Read the model definition and answer for the solid it produces. Units are mm, in the model's axes. Round coordinates to 2 decimals unless told otherwise and drop trailing zeros. Order: outer loops, then holes, each group sorted by start corner. A loop starts at its lowest first (then second) coordinate and runs counter-clockwise, first axis right, second up. Notation, with made-up numbers: M -7,7 L 9,7 A18 cw 9,12 Z; hole C -12.5,23.25 d1. An arc over 180 degrees is marked long. Use one line per item in the form item = value. Start each with the question number.
Autodesk Inventor part; units mm, degrees
ref_plane "YZ Plane" through (0, 0, 0) normal (1, 0, 0) x (0, 1, 0)
ref_plane "XZ Plane" through (0, 0, 0) normal (0, 1, 0) x (-1, 0, 0)
ref_plane "XY Plane" through (0, 0, 0) normal (0, 0, 1) x (1, 0, 0)
sketch "Sketch1" plane through (0, 0, 0) normal (0, 0, 1) x (1, 0, 0)
  line L0 (0, 0) -> (68.834, 0)
  line L1 (68.834, 0) -> (68.834, 89.027)
  line L2 (68.834, 89.027) -> (0, 89.027)
  line L3 (0, 89.027) -> (0, 0)
  dimension "d0" = 89.027
  dimension "d1" = 68.834
extrude "Extrusion1" add sketch "Sketch1" along normal blind 7.62
sketch "Sketch2" plane through (0, 0, 7.62) normal (0, 0, 1) x (1, 0, 0)
  line L0 (68.834, 89.027) -> (0, 89.027)
  line L1 (0, 89.027) -> (3.81, 89.027)
  line L2 (3.81, 89.027) -> (3.81, 85.216)
  line L3 (3.81, 85.216) -> (0, 85.216)
  line L4 (0, 85.216) -> (0, 89.027)
  circle A0 centre (3.81, 85.216) radius 1.0414
  line L5 (68.834, 89.027) -> (65.024, 89.027)
  line L6 (65.024, 89.027) -> (65.024, 85.216)
  line L7 (65.024, 85.216) -> (68.834, 85.216)
  line L8 (68.834, 85.216) -> (68.834, 89.027)
  circle A1 centre (65.024, 85.216) radius 1.0414
  line L9 (0, 0) -> (68.834, 0)
  line L10 (68.834, 0) -> (65.024, 0)
  line L11 (65.024, 0) -> (65.024, 3.8136)
  line L12 (65.024, 3.8136) -> (68.834, 3.8136)
  line L13 (68.834, 3.8136) -> (68.834, 0)
  circle A2 centre (65.024, 3.8136) radius 1.0414
  line L14 (0, 0) -> (3.81, 0)
  line L15 (3.81, 0) -> (3.81, 3.8136)
  line L16 (3.81, 3.8136) -> (0, 3.8136)
  line L17 (0, 3.8136) -> (0, 0)
  circle A3 centre (3.81, 3.8136) radius 1.0414
  dimension "d4" = 3.81
  dimension "d5" = 2.0828
  dimension "d6" = 3.81
  dimension "d7" = 2.0828
  dimension "d8" = 2.0828
  dimension "d9" = 2.0828
extrude "Extrusion2" cut sketch "Sketch2" against normal blind 7.62 contours A0 L3 L2 | L2 L3 A0
extrude "Extrusion3" cut sketch "Sketch2" against normal blind 7.62 contours A1 L7 L6 | L6 L7 A1
extrude "Extrusion4" cut sketch "Sketch2" against normal blind 7.62 contours A2 L12 L11 | L11 L12 A2
extrude "Extrusion5" cut sketch "Sketch2" against normal blind 7.62 contours A3 L16 L15 | L15 L16 A3
properties part number "arduinoCover"
Item 1: For a pull along Y with two mould halves and no side action, classify faces 1 (the flat face through (68.834, 44, 4)), 2 (the flat face through (34, 0, 4)), 3 (the cylindrical face through (65.584, 4.692, 3.863)) as pulls with the +Y half, pulls with the -Y half, needs draft (parallel to the pull), parting line crosses it, or undercut.
Item 2: Section A-A (x = 3.81) is taken. Write down the section's boundary in (y, z) (3 decimals), and give its area (3 significant figures).
Item 3: Find the intervals of material crossed by L1, parallel to X at y = 4, z = 2.75; L2, parallel to Y at x = 3.81, z = 3 (3 decimals), in increasing order. Write a range as [from, to].
The answers:
q1.face_1 = needs draft
q1.face_2 = pulls with the -Y half
q1.face_3 = undercut
q2.outline = M 0,0 L 2.772,0 L 2.772,7.62 L 0,7.62 Z; M 4.855,0 L 84.175,0 L 84.175,7.62 L 4.855,7.62 Z; M 86.257,0 L 89.027,0 L 89.027,7.62 L 86.257,7.62 Z
q2.area = 647 mm²
q3.L1 = [0, 2.79], [4.83, 64], [66.05, 68.83]
q3.L2 = [0, 2.772], [4.855, 84.175], [86.257, 89.027]
